Can you work these out from the drawing? Everything is in mm from the part's minimum corner. Give positions to 0.01 mm unless a question says otherwise; leave off trailing zeros. Order: outer loops, then holes, each group sorted by start corner. A loop starts at its lowest first (then second) coordinate and runs counter-clockwise, first axis right, second up. Notation, with made-up numbers: (31.5, 6) - (40.5, 6) arc R17 cw to (40.5, 29) - close; hole circle Ø6 at (34.25, -31.5). An arc over 180 degrees is marked (long way). One line per question, with ' | ' between items.
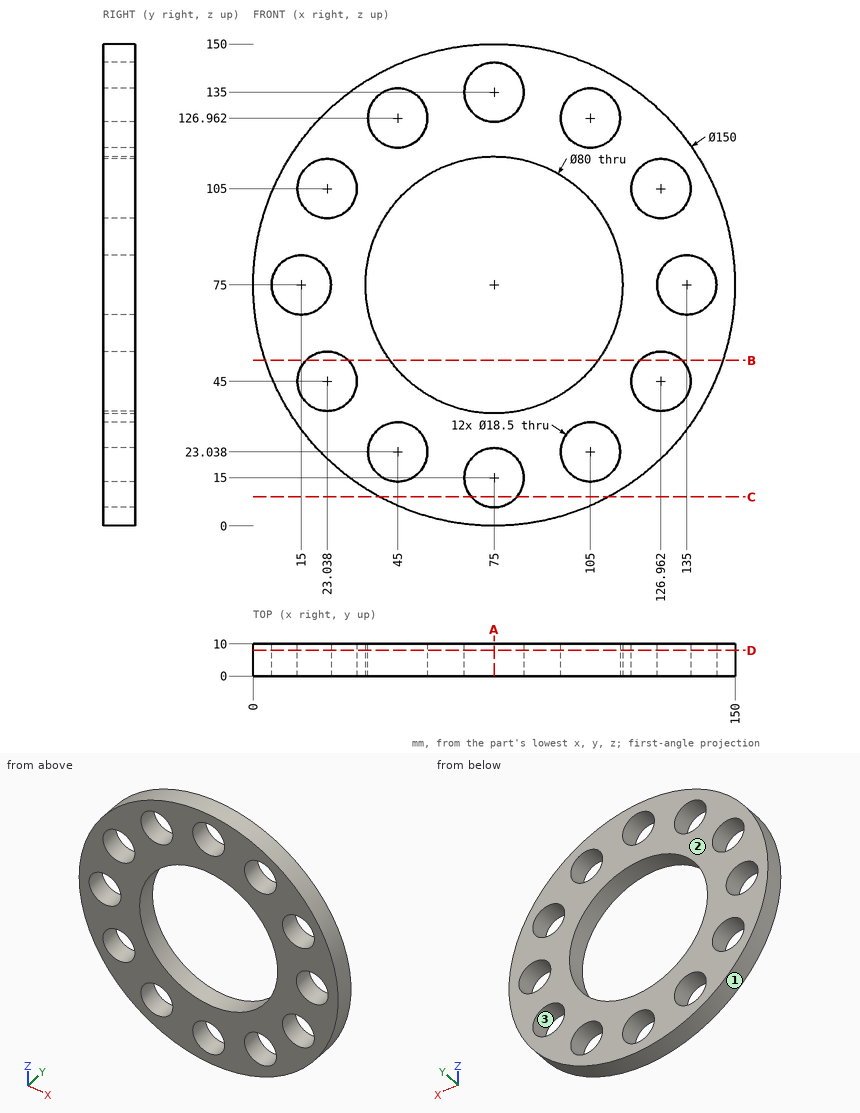
1) Please list where these lines run through material, in increasing order: L1, parallel to X at y = 2, z = 105 (1 decimal); L2, parallel to Z at x = 83, y = 1 (1 decimal); L3, parallel to X at y = 2, z = 47 (1 decimal).
Model answer:
L1: x = 6.3 to 13.8, 32.3 to 48.5, 101.5 to 117.7, 136.2 to 143.7 | L2: z = 0.4 to 10.4, 19.6 to 35.8, 114.2 to 130.4, 139.6 to 149.6 | L3: x = 5.4 to 14, 32.1 to 46.4, 103.6 to 117.9, 136 to 144.6
2) I want a section at A-A (x = 75). List the corners of the cut face in (y, z) for me, plus the area to 3 significant figures.
Model answer:
outline: (0, 0) - (10, 0) - (10, 5.75) - (0, 5.75) - close; (0, 24.25) - (10, 24.25) - (10, 35) - (0, 35) - close; (0, 115) - (10, 115) - (10, 125.75) - (0, 125.75) - close; (0, 144.25) - (10, 144.25) - (10, 150) - (0, 150) - close | area: 330 mm2
3) I want a section at C-C (z = 9). List the corners of the cut face in (x, y) for me.
Model answer:
outline: (39.38, 0) - (67.96, 0) - (67.96, 10) - (39.38, 10) - close; (82.04, 0) - (110.62, 0) - (110.62, 10) - (82.04, 10) - close
4) I want a section at D-D (y = 8). State how many separate pieces and enclosed holes the cut face has, plus the area to 3 significant figures.
Model answer:
separate pieces: 1 | enclosed holes: 13 | area: 9,420 mm2
5) I want a section at B-B (z = 51.5). List the corners of the cut face in (x, y) for me, plus the area to 3 significant figures.
Model answer:
outline: (3.78, 0) - (16.46, 0) - (16.46, 10) - (3.78, 10) - close; (29.62, 0) - (42.63, 0) - (42.63, 10) - (29.62, 10) - close; (107.37, 0) - (120.38, 0) - (120.38, 10) - (107.37, 10) - close; (133.54, 0) - (146.22, 0) - (146.22, 10) - (133.54, 10) - close | area: 514 mm2
6) Thinking about a two-plate mould opening in Z: for the marked faces 1, 2 and 3, which applies, +Z half, -Z half, draft (parallel to the pull), parting line (faces both ways), or undercut?
Model answer:
face 1: parting line | face 2: draft | face 3: undercut
7) I'm going to push flat-ended pins straight in: P1, Ø1.5, axis at x = 27.5, y = 7.5, coming from the +Z side (1 decimal); P2, Ø6, axis at x = 21.5, y = 2, coming from the +Z side; P3, Ø5, axis at x = 37.5, y = 2, coming from the -Z side. Where does each tip first touch, or does it pass through?
Model answer:
P1: stops at z = 133.6 | P2: stops at z = 130.45 | P3: stops at z = 8.67
